from build123d import *

# Parameters (mm, degrees)
SKETCH1_W                                       = 292.1
SKETCH1_H                                       = 50.8
BOSS_EXTRUDE1_DEPTH                             = 6.35
CBORE_FOR_10_SOCKET_HEAD_CAP_SCREW1_D           = 5.1054
CBORE_FOR_10_SOCKET_HEAD_CAP_SCREW1_CBORE_D     = 9.525
CBORE_FOR_10_SOCKET_HEAD_CAP_SCREW1_CBORE_DEPTH = 2.54
F_1_4_CLEARANCE_HOLE1_D                         = 6.7564
FILLET1_R                                       = 2.54
CUT_EXTRUDE1_DEPTH                              = 7.35


with BuildPart() as part:
    # Sketch1 → Boss-Extrude1 (new body)
    with BuildSketch(Plane(origin=(0, 0, 0), x_dir=(1, 0, 0), z_dir=(0, 1, 0))):
        Rectangle(SKETCH1_W, SKETCH1_H)
    extrude(amount=BOSS_EXTRUDE1_DEPTH)

    # CBORE for #10 Socket Head Cap Screw1 (through all)
    with Locations(Plane(origin=(0, 6.35, 0), x_dir=(1, 0, 0), z_dir=(0, 1, 0))):
        with Locations((44.45, 12.7), (6.35, 12.7), (6.35, -12.7), (44.45, -12.7), (-111.252, 12.7), (-111.252, 0), (-111.252, -12.7), (57.15, 12.7), (57.15, -12.7)):
            CounterBoreHole(CBORE_FOR_10_SOCKET_HEAD_CAP_SCREW1_D / 2, CBORE_FOR_10_SOCKET_HEAD_CAP_SCREW1_CBORE_D / 2, CBORE_FOR_10_SOCKET_HEAD_CAP_SCREW1_CBORE_DEPTH)

    # 1/4 Clearance Hole1 (through all)
    with Locations(Plane.XZ):
        with Locations((-136.525, 12.7), (-136.525, 0), (-136.525, -12.7), (136.525, 12.7), (136.525, 0), (136.525, -12.7)):
            Hole(F_1_4_CLEARANCE_HOLE1_D / 2)

    # Fillet1
    fillet1_edges = [part.edges().sort_by_distance(p)[0] for p in [
        (146.05, 3.175, 25.4),
        (-146.05, 3.175, 25.4),
        (-146.05, 3.175, -25.4),
        (146.05, 3.175, -25.4),
    ]]
    fillet(fillet1_edges, radius=FILLET1_R)

    # Sketch8 → Cut-Extrude1 (cut, through all)
    with BuildSketch(Plane.XZ):
        with BuildLine():
            Line((-83.502395687, -19.05), (-21.399604313, -19.05))
            ThreePointArc((-21.399604313, -19.05), (-19.407898045, -17.420653874), (-20.61026549, -15.145576911))
            Line((-20.61026549, -15.145576911), (-51.661661177, -2.055548129))
            ThreePointArc((-51.661661177, -2.055548129), (-52.451, -1.895971218), (-53.240338823, -2.055548129))
            Line((-53.240338823, -2.055548129), (-84.29173451, -15.145576911))
            ThreePointArc((-84.29173451, -15.145576911), (-85.494101955, -17.420653874), (-83.502395687, -19.05))
        make_face()
        with BuildLine():
            Line((-101.727, -15.988213098), (-101.727, 15.988213098))
            ThreePointArc((-101.727, 15.988213098), (-100.818629724, 17.681281391), (-98.905661177, 17.860636186))
            Line((-98.905661177, 17.860636186), (-60.979363267, 1.872423089))
            ThreePointArc((-60.979363267, 1.872423089), (-59.73670209, 0), (-60.979363267, -1.872423089))
            Line((-60.979363267, -1.872423089), (-98.905661177, -17.860636186))
            ThreePointArc((-98.905661177, -17.860636186), (-100.818629724, -17.681281391), (-101.727, -15.988213098))
        make_face()
        with BuildLine():
            Line((-83.502395687, 19.05), (-21.399604313, 19.05))
            ThreePointArc((-21.399604313, 19.05), (-19.407898045, 17.420653874), (-20.61026549, 15.145576911))
            Line((-20.61026549, 15.145576911), (-51.661661177, 2.055548129))
            ThreePointArc((-51.661661177, 2.055548129), (-52.451, 1.895971218), (-53.240338823, 2.055548129))
            Line((-53.240338823, 2.055548129), (-84.29173451, 15.145576911))
            ThreePointArc((-84.29173451, 15.145576911), (-85.494101955, 17.420653874), (-83.502395687, 19.05))
        make_face()
        with BuildLine():
            Line((-3.175, -15.988213098), (-3.175, 15.988213098))
            ThreePointArc((-3.175, 15.988213098), (-4.083370276, 17.681281391), (-5.996338823, 17.860636186))
            Line((-5.996338823, 17.860636186), (-43.922636733, 1.872423089))
            ThreePointArc((-43.922636733, 1.872423089), (-45.16529791, 0), (-43.922636733, -1.872423089))
            Line((-43.922636733, -1.872423089), (-5.996338823, -17.860636186))
            ThreePointArc((-5.996338823, -17.860636186), (-4.083370276, -17.681281391), (-3.175, -15.988213098))
        make_face()
        with BuildLine():
            Line((20.455368131, -16.247256429), (31.012846191, 9.506682143))
            ThreePointArc((31.012846191, 9.506682143), (33.285779492, 10.729615644), (34.925, 8.735938572))
            Line((34.925, 8.735938572), (34.925, -17.018))
            ThreePointArc((34.925, -17.018), (34.329840979, -18.454840979), (32.893, -19.05))
            Line((32.893, -19.05), (22.33552194, -19.05))
            ThreePointArc((22.33552194, -19.05), (20.64804232, -18.150005535), (20.455368131, -16.247256429))
        make_face()
        with BuildLine():
            Line((15.875, -8.735938572), (15.875, 17.018))
            ThreePointArc((15.875, 17.018), (16.470159021, 18.454840979), (17.907, 19.05))
            Line((17.907, 19.05), (28.46447806, 19.05))
            ThreePointArc((28.46447806, 19.05), (30.15195768, 18.150005535), (30.344631869, 16.247256429))
            Line((30.344631869, 16.247256429), (19.787153809, -9.506682143))
            ThreePointArc((19.787153809, -9.506682143), (17.514220508, -10.729615644), (15.875, -8.735938572))
        make_face()
        with BuildLine():
            Line((78.713510728, -19.05), (114.961489272, -19.05))
            ThreePointArc((114.961489272, -19.05), (116.900367087, -17.626092773), (116.121939653, -15.349953564))
            Line((116.121939653, -15.349953564), (97.997950381, -2.741197719))
            ThreePointArc((97.997950381, -2.741197719), (96.8375, -2.377244155), (95.677049619, -2.741197719))
            Line((95.677049619, -2.741197719), (77.553060347, -15.349953564))
            ThreePointArc((77.553060347, -15.349953564), (76.774632913, -17.626092773), (78.713510728, -19.05))
        make_face()
        with BuildLine():
            Line((66.675, -15.160984063), (66.675, 15.160984063))
            ThreePointArc((66.675, 15.160984063), (67.765992873, 16.961964237), (69.867450381, 16.8290305))
            Line((69.867450381, 16.8290305), (91.660045614, 1.668046436))
            ThreePointArc((91.660045614, 1.668046436), (92.531595233, 0), (91.660045614, -1.668046436))
            Line((91.660045614, -1.668046436), (69.867450381, -16.8290305))
            ThreePointArc((69.867450381, -16.8290305), (67.765992873, -16.961964237), (66.675, -15.160984063))
        make_face()
        with BuildLine():
            Line((78.713510728, 19.05), (114.961489272, 19.05))
            ThreePointArc((114.961489272, 19.05), (116.900367087, 17.626092773), (116.121939653, 15.349953564))
            Line((116.121939653, 15.349953564), (97.997950381, 2.741197719))
            ThreePointArc((97.997950381, 2.741197719), (96.8375, 2.377244155), (95.677049619, 2.741197719))
            Line((95.677049619, 2.741197719), (77.553060347, 15.349953564))
            ThreePointArc((77.553060347, 15.349953564), (76.774632913, 17.626092773), (78.713510728, 19.05))
        make_face()
        with BuildLine():
            Line((127, -15.160984063), (127, 15.160984063))
            ThreePointArc((127, 15.160984063), (125.909007127, 16.961964237), (123.807549619, 16.8290305))
            Line((123.807549619, 16.8290305), (102.014954386, 1.668046436))
            ThreePointArc((102.014954386, 1.668046436), (101.143404767, 0), (102.014954386, -1.668046436))
            Line((102.014954386, -1.668046436), (123.807549619, -16.8290305))
            ThreePointArc((123.807549619, -16.8290305), (125.909007127, -16.961964237), (127, -15.160984063))
        make_face()
    extrude(amount=-CUT_EXTRUDE1_DEPTH, mode=Mode.SUBTRACT)


solid = part.part
Can you work these out from the model? Positions are in its coordinate system, mm. A direction names the side the tool comes from. Give positions to 0.01 mm unless a question says otherwise; leave off trailing zeros. Loops run counter-clockwise (first coordinate to the right, second up) from the corner with the lowest first, then second, coordinate; pieces in that order, holes last. Notation, with made-up numbers: (0.25, 87) -> (15.25, 87) arc R29 ccw to (15.25, 120) -> close; hole circle Ø8 at (-40, 16). An arc over 180 degrees is marked (long way). Write item = value, one per line.
1) Suppose I cut it at B-B on y = 5.25. Give the number of separate pieces and of enclosed holes in the cut face, then the cut area to 3 significant figures.
Check result:
separate_pieces = 1
enclosed_holes = 25
area = 8,510 mm2
2) I need wall thicknesses on L1, parallel to Z at x = 6.35, y = 1.8; L2, parallel to Z at x = 85, y = 5.5. Which ranges of each line are inside material? Lowest first, please. Write a range as from..to.
Check result:
L1 = -25.4..-15.25, -10.15..10.15, 15.25..25.4
L2 = -25.4..-19.05, -10.17..-6.3, 6.3..10.17, 19.05..25.4
3) Will these pins go through, and if not, where does the flat tip stop? pin 1 (5 mm diameter, centred on x = 46.5, z = -13, fed in from +Y); pin 2 (5.5 mm diameter, centred on x = -136.525, z = 12.7, fed in from +Y).
Check result:
pin_1 = 3.81
pin_2 = through
4) Thinking about a two-plate mould opening in Z: for faces 1 (the cylindrical face through (-113.6, 1.9, -11.7)), 2 (the flat face through (-2, 0, 0)), which applies, released by +Z, released by -Z, zero draft, split by the parting line, or undercut?
Check result:
face_1 = undercut
face_2 = zero draft
5) Suppose I cut it at A-A on x = 6.35. Write out the boundary of the cut face in (y, z), then the cut area to 3 significant figures.
Check result:
outline = (0, -25.4) -> (6.35, -25.4) -> (6.35, -17.46) -> (3.81, -17.46) -> (3.81, -15.25) -> (0, -15.25) -> close; (0, -10.15) -> (3.81, -10.15) -> (3.81, -7.94) -> (6.35, -7.94) -> (6.35, 7.94) -> (3.81, 7.94) -> (3.81, 10.15) -> (0, 10.15) -> close; (0, 15.25) -> (3.81, 15.25) -> (3.81, 17.46) -> (6.35, 17.46) -> (6.35, 25.4) -> (0, 25.4) -> close
area = 235 mm2
6) Suppose I cut it at C-C on x = -89. Write out the boundary of the cut face in (y, z), then the cut area to 3 significant figures.
Check result:
outline = (0, -25.4) -> (6.35, -25.4) -> (6.35, -13.68) -> (0, -13.68) -> close; (0, 13.68) -> (6.35, 13.68) -> (6.35, 25.4) -> (0, 25.4) -> close
area = 149 mm2
7) For faces 3 (the flat face through (23, 3, 19.05)), 4 (the cylindrical face through (5.73, 5.1, 7.98)), which set-ups out of +Z, -Z, +X, -X, +Y, -Y let a thin tool reach every point of the face, with its end or its side?
Check result:
face_3 = +Y, -Y
face_4 = +Y
